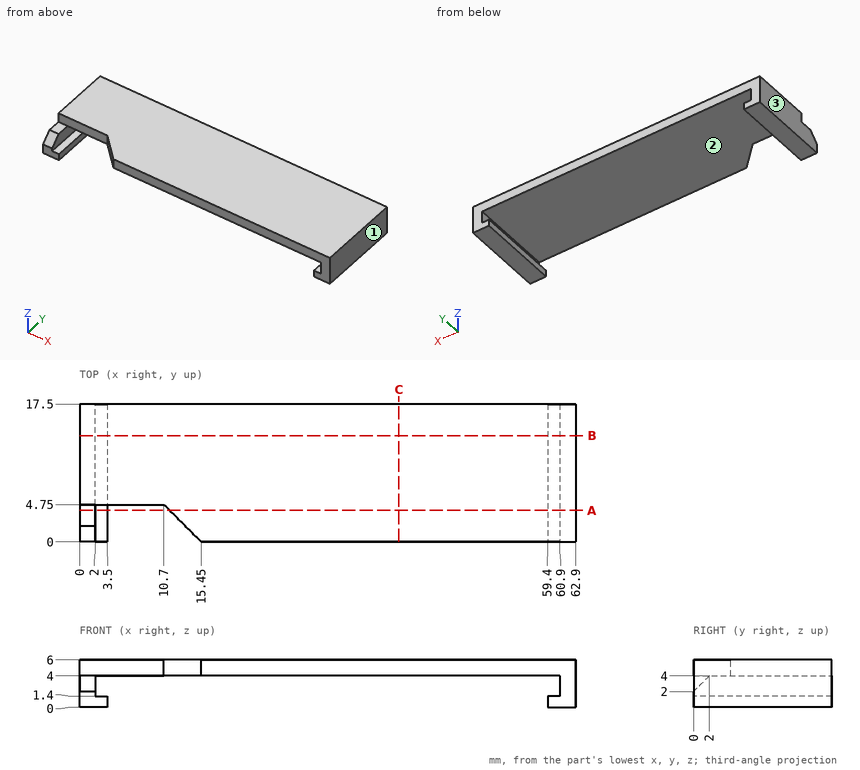
Job drawing, mm, ordinate dimensions from the low corner. One solid piece. Coordinates: 2 decimals unless noted, no trailing zeros. Write each loop counter-clockwise with the first axis right and the second up, starting at its lowest first coordinate (ties: lowest second). Pieces come first, ordered by that corner, then holes. Notation, with made-up numbers: (-31.5, 73.25) - (14.5, 73.25) arc R33 cw to (14.5, 110.25) - close; hole circle Ø10 at (54, 72). An arc over 180 degrees is marked (long way). Use a Markdown table: item, result. Add a question column.
Item 1: Band-saw the part on B-B, the plane y = 13.5. Give the cut face in (x, z).
Item 2: Flat gauge pins, fed straight in: pin 1 (0.6 mm diameter, centred on x = 1, y = 3.5, fed in from +Z); pin 2 (9 mm diameter, centred on x = 41, y = 11.5, fed in from -Z); pin 3 (1.6 mm diameter, centred on x = 6.5, z = 5, fed in from -Y); pin 4 (2 mm diameter, centred on x = 19.5, z = 2.5, fed in from +Y). Where does each tip first touch, or does it go through?
Item 3: Band-saw the part on A-A, the plane y = 4. Give the cut face in (x, z).
Item 4: Band-saw the part on C-C, the plane x = 40.5. Give the cut face in (y, z).
Item 5: Drill centre lines: L1, parallel to X at y = 4.75, z = 3.85; L2, parallel to X at y = 16.25, z = 1.1; L3, parallel to Z at x = 53, y = 6. Where is each one in solid material? Low to high. Write a range as from..to.
Item 6: Mould opens along X. For the marked faces 1, 2 and 3 say: pulls with the +X half, pulls with the -X half, needs draft (parallel to the pull), parting line crosses it, or undercut.
Numbers:
| question | item | result |
|---|---|---|
| 1 | outline | (0, 0) - (3.5, 0) - (3.5, 1.4) - (2, 1.4) - (2, 4) - (60.9, 4) - (60.9, 1.4) - (59.4, 1.4) - (59.4, 0) - (62.9, 0) - (62.9, 6) - (0, 6) - close |
| 2 | pin 1 | z = 4 |
| 2 | pin 2 | z = 4 |
| 2 | pin 3 | y = 4.75 |
| 2 | pin 4 | through |
| 3 | outline | (0, 0) - (3.5, 0) - (3.5, 1.4) - (2, 1.4) - (2, 4) - (0, 4) - close; (11.45, 4) - (60.9, 4) - (60.9, 1.4) - (59.4, 1.4) - (59.4, 0) - (62.9, 0) - (62.9, 6) - (11.45, 6) - close |
| 4 | outline | (0, 4) - (17.5, 4) - (17.5, 6) - (0, 6) - close |
| 5 | L1 | 0..2, 60.9..62.9 |
| 5 | L2 | 0..3.5, 59.4..62.9 |
| 5 | L3 | 4..6 |
| 6 | face 1 | pulls with the +X half |
| 6 | face 2 | undercut |
| 6 | face 3 | pulls with the -X half |
